Verification items for the finished model (mm, model axes). A direction names the side the tool comes from. Coordinates: 2 decimals unless noted, no trailing zeros. Order: outer loops, then holes, each group sorted by start corner. A loop starts at its lowest first (then second) coordinate and runs counter-clockwise, first axis right, second up. Notation, with made-up numbers: M 2.5,33.5 L 21.5,33.5 A24 ccw 21.5,52.5 Z; hole C 89,8 d4. An arc over 180 degrees is marked long. Write item = value, one per line.
```python
from build123d import *

# Parameters (mm, degrees)
BOSS_EXTRUDE2_DEPTH = 1200
SKETCH2_R           = 25
SKETCH2_R_2         = 10
CUT_EXTRUDE1_DEPTH  = 1200


with BuildPart() as part:
    # Sketch1 → Boss-Extrude2 (new body)
    with BuildSketch(Plane(origin=(0, 0, 0), x_dir=(0, 0, -1), z_dir=(1, 0, 0))):
        Polygon((-25, 75), (-25, 85), (35, 85), (35, -85), (-25, -85), (-25, -75), (25, -75), (25, 75), align=None)
    extrude(amount=BOSS_EXTRUDE2_DEPTH)

    # Sketch2 → Cut-Extrude1 (cut)
    with BuildSketch(Plane.XY.offset(-25)):
        with Locations((1000, 0)):
            Circle(SKETCH2_R)
        with Locations((950, 0)):
            Circle(SKETCH2_R_2)
        with Locations((1000, 50)):
            Circle(SKETCH2_R_2)
        with Locations((1000, -50)):
            Circle(SKETCH2_R_2)
        with Locations((1050, 0)):
            Circle(SKETCH2_R_2)
    cut_extrude1 = extrude(amount=-CUT_EXTRUDE1_DEPTH, mode=Mode.SUBTRACT)

    # Mirror2: Cut-Extrude1 across plane
    add(cut_extrude1.mirror(Plane(origin=(600, 0, 0), x_dir=(0, 0, 1), z_dir=(1, 0, 0))), mode=Mode.SUBTRACT)


solid = part.part
```
Item 1: Sectioned sample at D-D, the plane z = 10.5. Enter the section's corners in (x, y).
Report:
outline = M 0,-85 L 1200,-85 L 1200,-75 L 0,-75 Z; M 0,75 L 1200,75 L 1200,85 L 0,85 Z
Item 2: Sectioned sample at A-A, the plane x = 1050. Enter the section's corners in (y, z).
Report:
outline = M -85,-35 L -10,-35 L -10,-25 L -75,-25 L -75,25 L -85,25 Z; M 10,-35 L 85,-35 L 85,25 L 75,25 L 75,-25 L 10,-25 Z
Item 3: Tool access check on faces 1 (the cylindrical face through (240.763, -3.83, -29.93)), 2 (the flat face through (592, -1, -25)). Record the directions out of +Z, -Z, +X, -X, +Y, -Y that give a thin tool (end or side, any length) a straight path to the whole face; none if there is none.
Report:
face_1 = +Z, -Z
face_2 = +Z, +X, -X
Item 4: Scan lines: L1, parallel to Y at x = 200, z = -31; L2, parallel to Y at x = 276.5, z = -15.5; L3, parallel to Y at x = 150, z = -26.75. Record each from-to range of solid material in increasing order. Write a range as from..to.
Report:
L1 = -85..-60, -40..-25, 25..40, 60..85
L2 = -85..-75, 75..85
L3 = -85..-10, 10..85
Item 5: Gauge pin test, flat end, axial feed: pin 1 (1 mm diameter, centred on x = 229.5, y = -49, fed in from +Z). Record the tip position at first contact, or that the pin passes through.
Report:
pin_1 = -25
Item 6: Sectioned sample at B-B, the plane y = -50. Enter the section's corners in (x, z).
Report:
outline = M 0,-35 L 190,-35 L 190,-25 L 0,-25 Z; M 210,-35 L 990,-35 L 990,-25 L 210,-25 Z; M 1010,-35 L 1200,-35 L 1200,-25 L 1010,-25 Z
Item 7: Sectioned sample at C-C, the plane x = 200. Enter the section's corners in (y, z), then the cut area to 3 significant figures.
Report:
outline = M -85,-35 L -60,-35 L -60,-25 L -75,-25 L -75,25 L -85,25 Z; M -40,-35 L -25,-35 L -25,-25 L -40,-25 Z; M 25,-35 L 40,-35 L 40,-25 L 25,-25 Z; M 60,-35 L 85,-35 L 85,25 L 75,25 L 75,-25 L 60,-25 Z
area = 1,800 mm^2
Item 8: Release check for a two-part mould opening along Y. For faces 3 (the flat face through (592, -85, -5)), 4 (the cylindrical face through (140.763, -3.83, -29.93)), 5 (the flat face through (592, 1, -35)) record: pulls with the +Y half, pulls with the -Y half, needs draft (parallel to the pull), parting line crosses it, or undercut.
Report:
face_3 = pulls with the -Y half
face_4 = undercut
face_5 = needs draft
